Read the model definition and answer for the solid it produces. Units are mm, in the model's axes. Face numbers are marked on the shaded views. A direction names the side the tool comes from. Coordinates: 2 decimals unless noted, no trailing zeros. Loops run counter-clockwise (first coordinate to the right, second up) from the corner with the lowest first, then second, coordinate; pieces in that order, holes last.
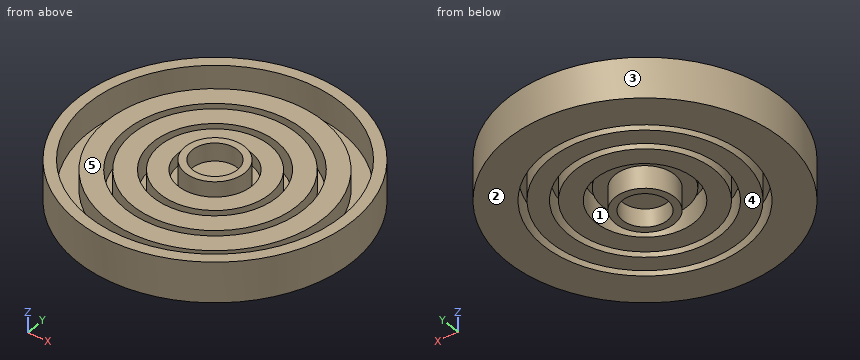
from build123d import *

# Parameters (mm, degrees)
F0_W   = 6.25
F0_H   = 2
F0_W_2 = 2
F0_H_2 = 0.75
F0_H_3 = 1.5
F0_W_3 = 5
F0_H_4 = 3


with BuildPart() as f2:
    # F0 (on Front) → F2 (revolve)
    with BuildSketch(Plane.XZ):
        with Locations((3.125, 1)):
            Rectangle(F0_W, F0_H)
        with Locations((3.125, -1)):
            Rectangle(F0_W, F0_H)
        Polygon((8.25, 0), (6.25, 0), (6.25, -2), (6.25, -7), (8.25, -7), (8.25, -0.75), align=None)
        Polygon((6.25, 2), (6.25, 0), (8.25, 0), (8.25, 0.75), (8.25, 7), (6.25, 7), align=None)
        with Locations((9.25, -0.375)):
            Rectangle(F0_W_2, F0_H_2)
        with Locations((9.25, 0.375)):
            Rectangle(F0_W_2, F0_H_2)
        Polygon((10.25, 0.75), (10.25, 0), (10.25, -0.75), (11.75, -0.75), (11.75, 2.75), (11.75, 4.25), (10.25, 4.25), align=None)
        with Locations((12.75, 3.5)):
            Rectangle(F0_W_2, F0_H_3)
        Polygon((15.25, 4.25), (13.75, 4.25), (13.75, 2.75), (13.75, -4.25), (15.25, -4.25), (15.25, -2.75), align=None)
        with Locations((16.25, -3.5)):
            Rectangle(F0_W_2, F0_H_3)
        Polygon((17.25, 4.25), (17.25, -2.75), (17.25, -4.25), (19.25, -4.25), (19.25, 2.75), (19.25, 4.25), align=None)
        with Locations((20.25, 3.5)):
            Rectangle(F0_W_2, F0_H_3)
        Polygon((22.75, 4.25), (21.25, 4.25), (21.25, 2.75), (21.25, -4.25), (22.75, -4.25), (22.75, -2.75), align=None)
        with Locations((23.75, -3.5)):
            Rectangle(F0_W_2, F0_H_3)
        Polygon((24.75, 4.25), (24.75, -2.75), (24.75, -4.25), (26.25, -4.25), (26.25, 2.75), (26.25, 4.25), align=None)
        with Locations((27.25, 3.5)):
            Rectangle(F0_W_2, F0_H_3)
        Polygon((30.25, 4.25), (28.25, 4.25), (28.25, 2.75), (28.25, -4.25), (30.25, -4.25), (30.25, -1.25), align=None)
        with Locations((32.75, -2.75)):
            Rectangle(F0_W_3, F0_H_4)
        Polygon((35.25, 7), (35.25, -1.25), (35.25, -4.25), (38.25, -4.25), (38.25, 7), align=None)
    revolve(axis=Axis((0, 0, -2.002694), (0, 0, -1)))


solid = f2.part
Item 1: A cutting plane is placed at A-A on z = 5.75. Determine the outline of the cut face in (x, y), then the cut area to 3 significant figures.
Numbers:
outline: circle Ø76.5 at (0, 0); circle Ø16.5 at (0, 0); hole circle Ø70.5 at (0, 0); hole circle Ø12.5 at (0, 0)
area: 784 mm2
Item 2: Find the intervals of material crossed by line 1 along Y through (x, z) = (0, 5.7); line 2 along Z through (x, y) = (12, -34); line 3 along Z through (x, y) = (-15, 5), in increasing order.
Numbers:
line 1: y = -38.25 to -35.25, -8.25 to -6.25, 6.25 to 8.25, 35.25 to 38.25
line 2: z = -4.25 to 7
line 3: z = -4.25 to -2.75
Item 3: Given pin 1 (1.5 mm diameter, centred on y = 23, z = -3, fed in from +X); pin 2 (1.5 mm diameter, centred on x = -13.5, z = 2, fed in from -Y); pin 3 (1 mm diameter, centred on x = 7.5, y = 14, fed in from +Z), each flat-ended and moving along its own axis, determine where each tip first touches the part or whether it passes through.
Numbers:
pin 1: stops at x = 31.11
pin 2: stops at y = -36.06
pin 3: stops at z = -2.75
Item 4: Which of the six approach directions +Z, -Z, +X, -X, +Y, -Y give full straight-line access (tool end or side, diameter ignored) to the marked faces 4 and 5?
Numbers:
face 4: -Z
face 5: +Z
Item 5: Determine the mould class of the marked faces 1, 2 and 3 for opening direction X: released by +X, released by -X, zero draft, split by the parting line, or undercut.
Numbers:
face 1: undercut
face 2: zero draft
face 3: split by the parting line
